from build123d import *

# Parameters (mm, degrees)
BOSS_EXTRUDE1_DEPTH     = 70
SKETCH3_R               = 3
CUT_EXTRUDE1_DEPTH      = 44
SKETCH7_R               = 7.5
CUT_EXTRUDE3_DEPTH      = 1
CUT_EXTRUDE3_DEPTH_BACK = 30
SKETCH5_W               = 15
SKETCH5_H               = 52
CUT_EXTRUDE2_DEPTH      = 5


with BuildPart() as part:
    # Sketch1 → Boss-Extrude1 (new body)
    with BuildSketch(Plane(origin=(0, 0, 0), x_dir=(1, 0, 0), z_dir=(0, 1, 0))):
        Polygon((-111.978184725, 0), (37.5, 0), (37.5, 43), (-37.5, 43), align=None)
    extrude(amount=BOSS_EXTRUDE1_DEPTH)

    # Sketch3 → Cut-Extrude1 (cut, through all)
    with BuildSketch(Plane.XY):
        with Locations((0, 18)):
            Circle(SKETCH3_R)
    extrude(amount=-CUT_EXTRUDE1_DEPTH, mode=Mode.SUBTRACT)

    # Sketch7 → Cut-Extrude3 (cut, two sides)
    with BuildSketch(Plane.XY) as cut_extrude3_sk:
        with Locations((0, 18)):
            Circle(SKETCH7_R)
    extrude(amount=CUT_EXTRUDE3_DEPTH, mode=Mode.SUBTRACT)
    extrude(cut_extrude3_sk.sketch, amount=-CUT_EXTRUDE3_DEPTH_BACK, mode=Mode.SUBTRACT)

    # Sketch5 → Cut-Extrude2 (cut)
    with BuildSketch(Plane.XY):
        with Locations((0, 44)):
            Rectangle(SKETCH5_W, SKETCH5_H)
    extrude(amount=-CUT_EXTRUDE2_DEPTH, mode=Mode.SUBTRACT)


solid = part.part
The listing builds one solid part. Answer for the finished solid, in the listing's coordinates (mm). A direction names the side the tool comes from. Coordinates: 2 decimals unless noted, no trailing zeros. Write each loop counter-clockwise with the first axis right and the second up, starting at its lowest first coordinate (ties: lowest second). Pieces come first, ordered by that corner, then holes. Notation, with made-up numbers: M -19,81.25 L 38,81.25 A22 ccw 38,112.25 Z; hole C -19,-8 d8. An arc over 180 degrees is marked long. Use one line per item in the form item = value.
Item 1: Given P1, Ø10, axis at x = -86.5, z = -16, coming from the -Y side; P2, Ø4, axis at y = 47, z = -3, coming from the -X side; P3, Ø7, axis at x = 0, y = 18, coming from the +Z side; P4, Ø8, axis at y = 33.5, z = -22, coming from the -X side, each flat-ended and moving along its own axis, determine where each tip first touches the part or whether it passes through.
Model answer:
P1 = 0
P2 = -110.25
P3 = -30
P4 = -80.8
Item 2: For faces 4 (the face through (-0.65, 15.07, -36.41)), 5 (the face through (-7.5, 44, -2)), 6 (the face through (3.2, 18.1, -30)), determine the directions among +Z, -Z, +X, -X, +Y, -Y from which every point of the face is accessible in a straight line to the end or side of a thin tool.
Model answer:
face_4 = +Z, -Z
face_5 = +Z, +Y
face_6 = +Z
Item 3: Find section A-A, the plane x = 0. Give the vertices of the cut face in (y, z).
Model answer:
outline = M 0,-43 L 15,-43 L 15,-30 L 10.5,-30 L 10.5,0 L 0,0 Z; M 21,-43 L 70,-43 L 70,-5 L 25.5,-5 L 25.5,-30 L 21,-30 Z
Item 4: Find section D-D, the plane z = -32. Give the vertices of the cut face in (x, y), plus the area to 3 significant figures.
Model answer:
outline = M -56.55,0 L 37.5,0 L 37.5,70 L -56.55,70 Z; hole C 0,18 d6
area = 6,560 mm2
Item 5: Find section B-B, the plane y = 60. Give the vertices of the cut face in (x, z), plus the area to 3 significant figures.
Model answer:
outline = M -111.98,0 L -37.5,-43 L 37.5,-43 L 37.5,0 L 7.5,0 L 7.5,-5 L -7.5,-5 L -7.5,0 Z
area = 4,750 mm2
Item 6: Find the intervals of material crossed by probe 1 along Y at (x, z) = (0, -35.5); probe 2 along Y at (x, z) = (0, -13.5); probe 3 along X at (y, z) = (55.5, -4), in increasing order.
Model answer:
probe_1 = 0 to 15, 21 to 70
probe_2 = 0 to 10.5, 25.5 to 70
probe_3 = -105.05 to -7.5, 7.5 to 37.5
Item 7: The mould has two halves that part along Y. Classify faces 1 (the face through (-1.63, 10.68, -14.79)), 2 (the face through (-22, 70, -22)), 3 (the face through (7.5, 44, -2)): released by +Y, released by -Y, zero draft, split by the parting line, or undercut.
Model answer:
face_1 = undercut
face_2 = released by +Y
face_3 = zero draft
Item 8: Find section C-C, the plane z = -12.5. Give the vertices of the cut face in (x, y), plus the area to 3 significant figures.
Model answer:
outline = M -90.33,0 L 37.5,0 L 37.5,70 L -90.33,70 Z; hole C 0,18 d15
area = 8,770 mm2
